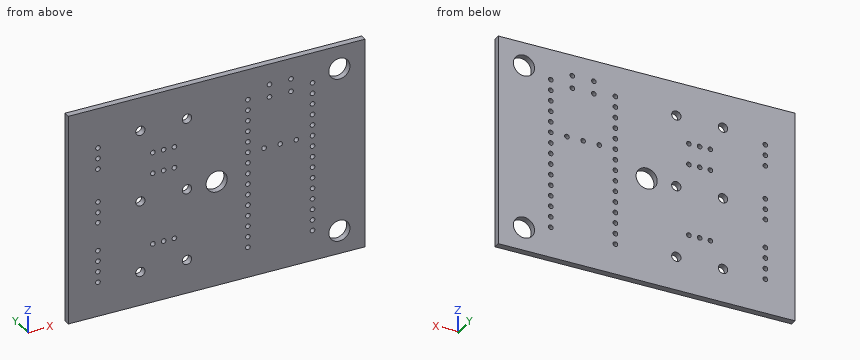
from build123d import *

# Parameters (mm, degrees)
SKETCH1_W           = 70
SKETCH1_H           = 50
BOSS_EXTRUDE1_DEPTH = 1.5
SKETCH2_R           = 2.5
CUT_EXTRUDE1_DEPTH  = 2.5
SKETCH4_R           = 1.1
SKETCH4_R_2         = 0.55
CUT_EXTRUDE2_DEPTH  = 2.5


with BuildPart() as part:
    # Sketch1 → Boss-Extrude1 (new body)
    with BuildSketch(Plane(origin=(0, 0, 0), x_dir=(1, 0, 0), z_dir=(0, 1, 0))):
        Rectangle(SKETCH1_W, SKETCH1_H)
    extrude(amount=BOSS_EXTRUDE1_DEPTH)

    # Sketch2 → Cut-Extrude1 (cut, through all)
    with BuildSketch(Plane(origin=(0, 1.5, 0), x_dir=(1, 0, 0), z_dir=(0, 1, 0))):
        Circle(SKETCH2_R)
        with Locations((28.95, 19.5)):
            Circle(SKETCH2_R)
        with Locations((28.95, -19.5)):
            Circle(SKETCH2_R)
    extrude(amount=-CUT_EXTRUDE1_DEPTH, mode=Mode.SUBTRACT)

    # Sketch4 → Cut-Extrude2 (cut, through all)
    with BuildSketch(Plane(origin=(0, 1.5, 0), x_dir=(1, 0, 0), z_dir=(0, 1, 0))):
        with Locations((-18, 0)):
            Circle(SKETCH4_R)
        with Locations((-7, 0)):
            Circle(SKETCH4_R)
        with Locations((-12.5, -6)):
            Circle(SKETCH4_R_2)
        with Locations((-9.96, -6)):
            Circle(SKETCH4_R_2)
        with Locations((-15.04, -6)):
            Circle(SKETCH4_R_2)
        with Locations((-12.5, 11)):
            Circle(SKETCH4_R_2)
        with Locations((-9.96, 11)):
            Circle(SKETCH4_R_2)
        with Locations((-15.04, 11)):
            Circle(SKETCH4_R_2)
        with Locations((-18, 17)):
            Circle(SKETCH4_R)
        with Locations((-7, 17)):
            Circle(SKETCH4_R)
        with Locations((-18, -17)):
            Circle(SKETCH4_R)
        with Locations((-7, -17)):
            Circle(SKETCH4_R)
        with Locations((7.38, 0)):
            Circle(SKETCH4_R_2)
        with Locations((22.62, 0)):
            Circle(SKETCH4_R_2)
        with Locations((7.38, 2.54)):
            Circle(SKETCH4_R_2)
        with Locations((7.38, 5.08)):
            Circle(SKETCH4_R_2)
        with Locations((7.38, 7.62)):
            Circle(SKETCH4_R_2)
        with Locations((7.38, 10.16)):
            Circle(SKETCH4_R_2)
        with Locations((7.38, 12.7)):
            Circle(SKETCH4_R_2)
        with Locations((7.38, 15.24)):
            Circle(SKETCH4_R_2)
        with Locations((7.38, 17.78)):
            Circle(SKETCH4_R_2)
        with Locations((22.62, 2.54)):
            Circle(SKETCH4_R_2)
        with Locations((22.62, 5.08)):
            Circle(SKETCH4_R_2)
        with Locations((22.62, 7.62)):
            Circle(SKETCH4_R_2)
        with Locations((22.62, 10.16)):
            Circle(SKETCH4_R_2)
        with Locations((22.62, 12.7)):
            Circle(SKETCH4_R_2)
        with Locations((22.62, 15.24)):
            Circle(SKETCH4_R_2)
        with Locations((22.62, 17.78)):
            Circle(SKETCH4_R_2)
        with Locations((22.62, -17.78)):
            Circle(SKETCH4_R_2)
        with Locations((22.62, -15.24)):
            Circle(SKETCH4_R_2)
        with Locations((22.62, -12.7)):
            Circle(SKETCH4_R_2)
        with Locations((22.62, -10.16)):
            Circle(SKETCH4_R_2)
        with Locations((22.62, -7.62)):
            Circle(SKETCH4_R_2)
        with Locations((22.62, -5.08)):
            Circle(SKETCH4_R_2)
        with Locations((22.62, -2.54)):
            Circle(SKETCH4_R_2)
        with Locations((7.38, -17.78)):
            Circle(SKETCH4_R_2)
        with Locations((7.38, -15.24)):
            Circle(SKETCH4_R_2)
        with Locations((7.38, -12.7)):
            Circle(SKETCH4_R_2)
        with Locations((7.38, -10.16)):
            Circle(SKETCH4_R_2)
        with Locations((7.38, -7.62)):
            Circle(SKETCH4_R_2)
        with Locations((7.38, -5.08)):
            Circle(SKETCH4_R_2)
        with Locations((7.38, -2.54)):
            Circle(SKETCH4_R_2)
        with Locations((-28, -13)):
            Circle(SKETCH4_R_2)
        with Locations((-28, -10.46)):
            Circle(SKETCH4_R_2)
        with Locations((-28, -15.54)):
            Circle(SKETCH4_R_2)
        with Locations((-28, 11.73)):
            Circle(SKETCH4_R_2)
        with Locations((-28, 14.27)):
            Circle(SKETCH4_R_2)
        with Locations((-28, 9.19)):
            Circle(SKETCH4_R_2)
        with Locations((-28, 16.81)):
            Circle(SKETCH4_R_2)
        with Locations((-9.96, -11)):
            Circle(SKETCH4_R_2)
        with Locations((-12.5, -11)):
            Circle(SKETCH4_R_2)
        with Locations((-15.04, -11)):
            Circle(SKETCH4_R_2)
        with Locations((11.19, -5.08)):
            Circle(SKETCH4_R_2)
        with Locations((15, -5.08)):
            Circle(SKETCH4_R_2)
        with Locations((18.81, -5.08)):
            Circle(SKETCH4_R_2)
        with Locations((12.46, -20.08)):
            Circle(SKETCH4_R_2)
        with Locations((17.54, -20.08)):
            Circle(SKETCH4_R_2)
        with Locations((17.54, -17.08)):
            Circle(SKETCH4_R_2)
        with Locations((-28, 0)):
            Circle(SKETCH4_R_2)
        with Locations((-28, -2.54)):
            Circle(SKETCH4_R_2)
        with Locations((-28, 2.45)):
            Circle(SKETCH4_R_2)
        with Locations((12.46, -17.08)):
            Circle(SKETCH4_R_2)
    extrude(amount=-CUT_EXTRUDE2_DEPTH, mode=Mode.SUBTRACT)


solid = part.part
Could you check a few things on this model? Use its own coordinates, in mm. Coordinates: 2 decimals unless noted, no trailing zeros. Loops run counter-clockwise (first coordinate to the right, second up) from the corner with the lowest first, then second, coordinate; pieces in that order, holes last.
1. Imagine slicing it at A-A (x = 0). Please give me the cut outline in (y, z).
2. I need wall thicknesses on L1, parallel to Z at x = -15, y = 0.95; L2, parallel to X at y = 0.6, z = 15.24; L3, parallel to X at y = 0.35, z = -13. Which ranges of each line are inside material? Lowest first, please.
3. Imagine slicing it at B-B (x = -7). Please give me the cut outline in (y, z).
4. Imagine slicing it at C-C (y = 1.05). Give the number of separate pieces and of enclosed holes in the cut face, and give its area (3 significant figures).
Computed values:
1. outline: (0, -25) - (1.5, -25) - (1.5, -2.5) - (0, -2.5) - close; (0, 2.5) - (1.5, 2.5) - (1.5, 25) - (0, 25) - close
2. L1: z = -25 to -11.55, -10.45 to 5.45, 6.55 to 10.45, 11.55 to 25
2. L2: x = -35 to -28.46, -27.54 to 6.83, 7.93 to 22.07, 23.17 to 35
2. L3: x = -35 to 6.92, 7.84 to 22.16, 23.08 to 35
3. outline: (0, -25) - (1.5, -25) - (1.5, -18.1) - (0, -18.1) - close; (0, -15.9) - (1.5, -15.9) - (1.5, -1.1) - (0, -1.1) - close; (0, 1.1) - (1.5, 1.1) - (1.5, 15.9) - (0, 15.9) - close; (0, 18.1) - (1.5, 18.1) - (1.5, 25) - (0, 25) - close
4. separate pieces: 1
4. enclosed holes: 65
4. area: 3,370 mm2
